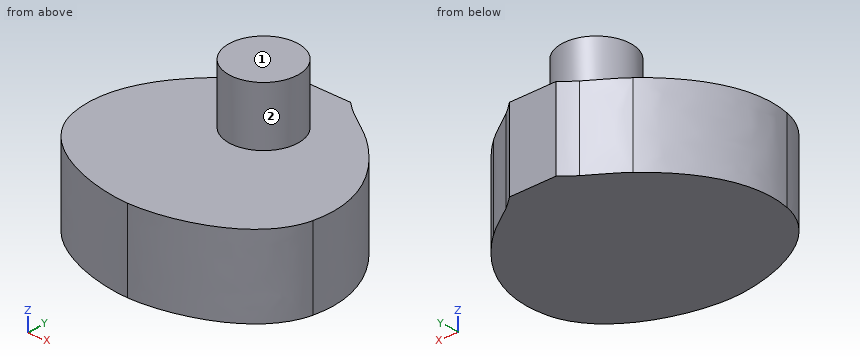
from build123d import *

# Parameters (mm, degrees)
SALIENTE_EXTRUIR1_DEPTH = 100
SALIENTE_EXTRUIR2_DEPTH = 100
CROQUIS13_R             = 42.623507313
SALIENTE_EXTRUIR3_DEPTH = 72


with BuildPart() as part:
    # Croquis1 → Saliente-Extruir1 (new body)
    with BuildSketch(Plane.XY):
        with BuildLine():
            Line((-28.560802162, 136.916395712), (2.54e-07, 136.916395712))
            Line((2.54e-07, 136.916395712), (2.54e-07, -136.916395712))
            add(Edge.make_bspline(
                [(2.54e-07, -136.916395712), (-46.441340442, -136.916395602), (-133.83340639, -111.670406771), (-147.578497366, -47.27649641)],
                knots=[0, 0, 0, 0, 1, 1, 1, 1], degree=3))
            add(Edge.make_bspline(
                [(-147.578497366, -47.27649641), (-163.110192587, 25.487257565), (-105.360717743, 78.580885367), (-85.639397682, 95.058759336)],
                knots=[0, 0, 0, 0, 1, 1, 1, 1], degree=3))
            add(Edge.make_bspline(
                [(-85.639397682, 95.058759336), (-70.778695882, 107.475422336), (-62.78576597, 110.83954464), (-45.323206026, 123.188624336)],
                knots=[0, 0, 0, 0, 1, 1, 1, 1], degree=3))
            add(Edge.make_bspline(
                [(-45.323206026, 123.188624336), (-39.50234289, 127.304974752), (-33.933522938, 132.194713512), (-28.560802162, 136.916395712)],
                knots=[0, 0, 0, 0, 1, 1, 1, 1], degree=3))
        make_face()
    extrude(amount=SALIENTE_EXTRUIR1_DEPTH)

    # Croquis3 → Saliente-Extruir2 (add)
    with BuildSketch(Plane.XY):
        with BuildLine():
            Line((2.54e-07, 136.916395712), (0, -136.916395712))
            add(Edge.make_bspline(
                [(0, -136.916395712), (46.441340696, -136.916395629), (133.833406659, -111.67040685), (147.578497673, -47.276496498)],
                knots=[0, 0, 0, 0, 1, 1, 1, 1], degree=3))
            add(Edge.make_bspline(
                [(147.578497673, -47.276496498), (163.110192997, 25.487257456), (105.360718228, 78.58088534), (85.63939819, 95.058759336)],
                knots=[0, 0, 0, 0, 1, 1, 1, 1], degree=3))
            add(Edge.make_bspline(
                [(85.63939819, 95.058759336), (70.77869639, 107.475422336), (62.785766478, 110.83954464), (45.323206534, 123.188624336)],
                knots=[0, 0, 0, 0, 1, 1, 1, 1], degree=3))
            add(Edge.make_bspline(
                [(45.323206534, 123.188624336), (39.502343398, 127.304974752), (33.933523446, 132.194713512), (28.56080267, 136.916395712)],
                knots=[0, 0, 0, 0, 1, 1, 1, 1], degree=3))
            Line((28.56080267, 136.916395712), (2.54e-07, 136.916395712))
        make_face()
    extrude(amount=SALIENTE_EXTRUIR2_DEPTH)

    # Croquis13 → Saliente-Extruir3 (add)
    with BuildSketch(Plane.XY.offset(100)):
        with Locations((2.54e-07, 49.659481629)):
            Circle(CROQUIS13_R)
    extrude(amount=SALIENTE_EXTRUIR3_DEPTH)


solid = part.part
Design review of the part built by this model. Coordinates are the model's own, in mm. Face numbers are marked on the shaded views. A direction names the side the tool comes from. Give positions to 0.01 mm unless a question says otherwise; leave off trailing zeros. Loops run counter-clockwise (first coordinate to the right, second up) from the corner with the lowest first, then second, coordinate; pieces in that order, holes last. Notation, with made-up numbers: (-9, 81) -> (4, 81) arc R20 ccw to (4, 88) -> close; hole circle Ø9 at (-1, 5.5). An arc over 180 degrees is marked (long way). One line per question, with ' | ' between items. Start each with the question number.
(1) For the marked faces 1 and 2, list the 3-axis set-ups (+Z, -Z, +X, -X, +Y, -Y) from which the entire face can be reached by the end or side of a thin tool; tool diameter is ignored.
(2) Insertion check: P1, Ø1.5, axis at x = 3.5, z = 153.5, coming from the -Y side; P2, Ø8, axis at y = 28.5, z = 137, coming from the +X side; P3, Ø1, axis at x = -94.5, y = 60, coming from the +Z side. Each pin has a flat end and moves straight along its axis. Give the tip position at first contact, or say it passes through.
(3) We need section A-A (z = 153.5). State the section outline as (x, y) points, and give its area (3 significant figures).
(4) For line 1 (Z direction, x = 19.5, y = -82); line 2 (Y direction, x = 26, z = 75.5); line 3 (X direction, y = -43.5, z = 69), list the stretches that pass through material, from the lowest coordinate up.
The answers:
1) face 1: +Z, +X, -X, +Y, -Y | face 2: +Z
2) P1: stops at y = 7.12 | P2: stops at x = 39.02 | P3: stops at z = 100
3) outline: circle Ø85.25 at (0, 49.66) | area: 5,710 mm^2
4) line 1: z = 0 to 100 | line 2: y = -134.76 to 136.92 | line 3: x = -148.32 to 148.32
